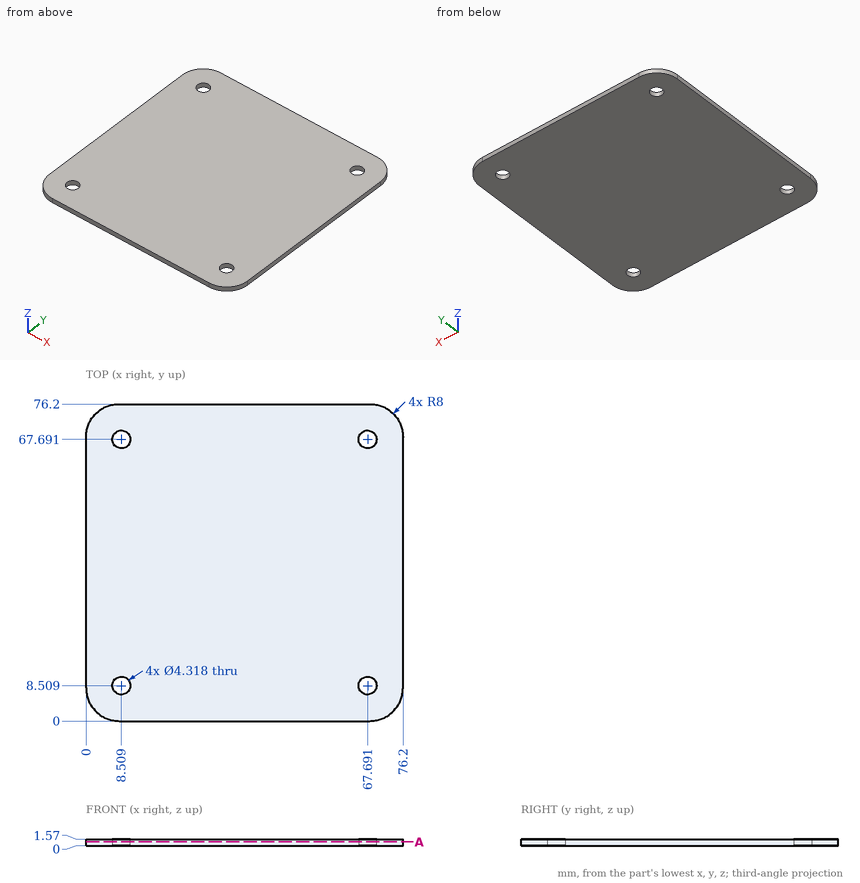
Design review of the part shown in the three views and the two pictorial views. Dimensions are in mm from the part's minimum x, y and z. Give positions to 0.01 mm unless a question says otherwise; leave off trailing zeros. Write each loop counter-clockwise with the first axis right and the second up, starting at its lowest first coordinate (ties: lowest second). Pieces come first, ordered by that corner, then holes. Notation, with made-up numbers: M -12,-26.5 L 9,-26.5 A21 cw 9,10.5 Z; hole C 55,53 d5. An arc over 180 degrees is marked long. Answer as CSV lines item,"result".
1. For pin 1 (4 mm diameter, centred on x = 67.691, y = 8.509, fed in from -Z), flat-tipped, find the tip position at first contact; note if it passes through.
Findings:
pin 1,"passes through"
2. Consider section A-A, the plane z = 0.85. Write out the cut boundary in (x, y).
Findings:
outline,"M 0,8 A8 ccw 8,0 L 68.2,0 A8 ccw 76.2,8 L 76.2,68.2 A8 ccw 68.2,76.2 L 8,76.2 A8 ccw 0,68.2 Z; hole C 8.51,8.51 d4.32; hole C 8.51,67.69 d4.32; hole C 67.69,8.51 d4.32; hole C 67.69,67.69 d4.32"
3. Wall thickness on line 1 (X direction, y = 69.5, z = 1.1); line 2 (X direction, y = 9, z = 1.35); line 3 (Y direction, x = 68.5, z = 0.85): over which ranges is each line inside the solid? List them lowest first.
Findings:
line 1,"x = 0.11 to 7.33, 9.69 to 66.51, 68.87 to 76.09"
line 2,"x = 0 to 6.41, 10.61 to 65.59, 69.79 to 76.2"
line 3,"y = 0.01 to 6.51, 10.51 to 65.69, 69.69 to 76.19"
